Can you work these out from the model? Positions are in its coordinate system, mm. A direction names the side the tool comes from. Give positions to 0.01 mm unless a question says otherwise; leave off trailing zeros. Order: outer loops, then holes, each group sorted by start corner. A loop starts at its lowest first (then second) coordinate and runs counter-clockwise, first axis right, second up. Notation, with made-up numbers: M -19.75,62 L 9.25,62 A6 ccw 9.25,66 Z; hole C 15,46.5 d2. An arc over 180 degrees is marked long. Use one line per item in the form item = value. Start each with the question number.
1. For faces 1 (the face through (257.361, 42, -6)), 2 (the face through (220, 177, 0)), which set-ups out of +Z, -Z, +X, -X, +Y, -Y let a thin tool reach every point of the face, with its end or its side?
2. I want a section at C-C, the plane x = 336.5. List the corners of the cut face in (y, z) for me (3 decimals), and give its area (3 significant figures).
3. I want a section at D-D, the plane y = 292.5. List the corners of the cut face in (x, z) for me.
4. I want a section at B-B, the plane z = -2.5. List the corners of the cut face in (x, y) for me (3 decimals).
5. We'd pull the mould along X, two halves only. Please class faces 3 (the face through (12.7, 172, -6)), 4 (the face through (487.99, 127.04, -6.26)), 5 (the face through (316, 61.056, -6)): +X half, -X half, draft (parallel to the pull), parting line (faces both ways), or undercut.
6. I need wall thicknesses on L1, parallel to X at y = 49, z = -10.25; L2, parallel to X at y = 44, z = -5.5; L3, parallel to Y at x = 285, z = -5.75 (3 decimals). Which ranges of each line are inside material? Lowest first, please.
7. I want a section at A-A, the plane x = 283. List the corners of the cut face in (y, z) for me (3 decimals), and give its area (3 significant figures).
8. Will these pins go through, and if not, where does the flat tip stop? P1, Ø4, axis at x = 238.5, z = -6, coming from the +Y side; P2, Ø1.5, axis at x = 173, z = -5.5, coming from the +Y side; P3, Ø6.5, axis at y = 44.5, z = -5.5, coming from the +X side.
```python
from build123d import *

# Parameters (mm, degrees)
BOSS_EXTRUDE1_DEPTH = 12.7
SKETCH2_W           = 117.66064382
SKETCH2_H           = 25.4
CUT_EXTRUDE1_DEPTH  = 13.7
FILLET1_R           = 12.7


with BuildPart() as part:
    # Sketch1 → Boss-Extrude1 (new body)
    with BuildSketch(Plane.XY):
        Polygon((12.7, 22.225), (12.7, 327.025), (536.089806585, 228.957542458), (438.52128764, 22.225), align=None)
    extrude(amount=-BOSS_EXTRUDE1_DEPTH)

    # Sketch2 → Cut-Extrude1 (cut, through all)
    with BuildSketch(Plane.XY):
        with Locations((147.73032191, 47.625)):
            Rectangle(SKETCH2_W, SKETCH2_H)
        with Locations((316.19096573, 48.355687107)):
            Rectangle(SKETCH2_W, SKETCH2_H)
    extrude(amount=-CUT_EXTRUDE1_DEPTH, mode=Mode.SUBTRACT)

    # Fillet1
    fillet1_edges = [part.edges().sort_by_distance(p)[0] for p in [
        (88.9, 60.325, -6.35),
        (206.56064382, 60.325, -6.35),
        (257.36064382, 61.055687107, -6.35),
        (375.02128764, 61.055687107, -6.35),
    ]]
    fillet(fillet1_edges, radius=FILLET1_R)


solid = part.part
```
Check result:
q1.face_1 = +Z, -Z
q1.face_2 = +Z, +X, -X, +Y, -Y
q2.outline = M 22.225,-12.7 L 35.656,-12.7 L 35.656,0 L 22.225,0 Z; M 61.056,-12.7 L 266.355,-12.7 L 266.355,0 L 61.056,0 Z
q2.area = 2,780 mm2
q3.outline = M 12.7,-12.7 L 196.96,-12.7 L 196.96,0 L 12.7,0 Z
q4.outline = M 12.7,22.225 L 438.521,22.225 L 536.09,228.958 L 12.7,327.025 Z; hole M 88.9,34.925 L 206.561,34.925 L 206.561,47.625 A12.7 ccw 193.861,60.325 L 101.6,60.325 A12.7 ccw 88.9,47.625 Z; hole M 257.361,35.656 L 375.021,35.656 L 375.021,48.356 A12.7 ccw 362.321,61.056 L 270.061,61.056 A12.7 ccw 257.361,48.356 Z
q5.face_3 = -X half
q5.face_4 = +X half
q5.face_5 = undercut
q6.L1 = 12.7 to 88.97, 206.49 to 257.38, 375 to 451.16
q6.L2 = 12.7 to 88.9, 206.56 to 257.36, 375.02 to 448.8
q6.L3 = 22.225 to 35.656, 61.056 to 276.004
q7.outline = M 22.225,-12.7 L 35.656,-12.7 L 35.656,0 L 22.225,0 Z; M 61.056,-12.7 L 276.379,-12.7 L 276.379,0 L 61.056,0 Z
q7.area = 2,910 mm2
q8.P1 = 285.09
q8.P2 = 297.13
q8.P3 = 450.57
